Work out the finished part from the listing and answer in its coordinate system (mm). Coordinates: 2 decimals unless noted, no trailing zeros. Order: outer loops, then holes, each group sorted by start corner. A loop starts at its lowest first (then second) coordinate and runs counter-clockwise, first axis right, second up. Notation, with made-up numbers: M 58,-40 L 73,-40 A21 cw 73,-21 Z; hole C 21.5,31 d4. An arc over 180 degrees is marked long. Answer in a Markdown table with one row per item. Add a question column.
Item 1: A flat-ended cylindrical pin translates along its axis: pin 1 Ø1 at (y, z) = (2, -2) entering from +X. Find the tip coordinate at first contact, or state that the pin passes through.
Item 2: The part is cut by section B-B (x = 1.3). Write down the section's boundary in (y, z), then the cut area to 3 significant figures.
Item 3: The mould has two halves that part along X. Classify faces 1 (the face through (0, 1, -2.598)), 2 (the face through (-2.242, 1.232, -1.314)), 3 (the face through (-1.71, 1.23, -0.38)), 4 (the face through (2.26, 1.23, -1.28)): released by +X, released by -X, zero draft, split by the parting line, or undercut.
Item 4: The part is cut by section A-A (z = 0). Write down the section's boundary in (x, y).
Item 5: Consider line 1 (X direction, y = 0.55, z = 0); line 2 (X direction, y = 2.05, z = -1.55); line 3 (Z direction, x = 2.3, y = 1.1). Determine where each line is inside the solid, lowest interval first. Write a range as from..to.
Item 6: The part is cut by section D-D (x = 1.95). Write down the section's boundary in (y, z), then the cut area to 3 significant figures.
Item 7: The part is cut by section C-C (y = 1.85). Write down the section's boundary in (x, z).
from build123d import *

# Parameters (mm, degrees)
SCHIZZO1_R                   = 1.75
ESTRUSIONE_ESTRUSIONE1_DEPTH = 2.5
RACCORDO1_R                  = 0.5


with BuildPart() as part:
    # Schizzo1 → Estrusione-Estrusione1 (new body)
    with BuildSketch(Plane(origin=(0, 0, 0), x_dir=(1, 0, 0), z_dir=(0, 1, 0))):
        Polygon((-1.5, 2.598076211), (-3, 0), (-1.5, -2.598076211), (1.5, -2.598076211), (3, 0), (1.5, 2.598076211), align=None)
        with Locations(Location((0, 0, 0), (0, 0, 270))):
            Circle(SCHIZZO1_R, mode=Mode.SUBTRACT)
    extrude(amount=ESTRUSIONE_ESTRUSIONE1_DEPTH)

    # Raccordo1
    raccordo1_edges = [part.edges().sort_by_distance(p)[0] for p in [
        (1.5, 1.25, -2.598076211),
        (3, 1.25, 0),
        (1.5, 1.25, 2.598076211),
        (-1.5, 1.25, 2.598076211),
        (-3, 1.25, 0),
        (-1.5, 1.25, -2.598076211),
    ]]
    fillet(raccordo1_edges, radius=RACCORDO1_R)


solid = part.part
Reply:
| question | item | result |
|---|---|---|
| 1 | pin 1 | stops at x = 2.13 |
| 2 | outline | M 0,-2.59 L 2.5,-2.59 L 2.5,-1.17 L 0,-1.17 Z; M 0,1.17 L 2.5,1.17 L 2.5,2.59 L 0,2.59 Z |
| 2 | area | 7.09 mm2 |
| 3 | face 1 | zero draft |
| 3 | face 2 | released by -X |
| 3 | face 3 | undercut |
| 3 | face 4 | released by +X |
| 4 | outline | M -2.92,0 L -1.75,0 L -1.75,2.5 L -2.92,2.5 Z; M 1.75,0 L 2.92,0 L 2.92,2.5 L 1.75,2.5 Z |
| 5 | line 1 | x = -2.92..-1.75, 1.75..2.92 |
| 5 | line 2 | x = -2.11..-0.81, 0.81..2.11 |
| 5 | line 3 | z = -1.21..1.21 |
| 6 | outline | M 0,-1.82 L 2.5,-1.82 L 2.5,1.82 L 0,1.82 Z |
| 6 | area | 9.09 mm2 |
| 7 | outline | M -2.86,-0.25 L -1.64,-2.35 A0.5 ccw -1.21,-2.6 L 1.21,-2.6 A0.5 ccw 1.64,-2.35 L 2.86,-0.25 A0.5 ccw 2.86,0.25 L 1.64,2.35 A0.5 ccw 1.21,2.6 L -1.21,2.6 A0.5 ccw -1.64,2.35 L -2.86,0.25 A0.5 ccw Z; hole C 0,0 d3.5 |
